from build123d import *

# Parameters (mm, degrees)
F1_DEPTH = 1750
F2_R     = 4
F3_R     = 2


with BuildPart() as f1:
    # F0 (on Front) → F1 (new body)
    with BuildSketch(Plane.XZ):
        Polygon((0, 0), (-20, 0), (-20, -10), (-10, -10), (-10, -75), (0, -75), align=None)
    extrude(amount=F1_DEPTH)

    # F2
    f2_edges = [f1.edges().sort_by_distance(p)[0] for p in [
        (0, -875, 0),
    ]]
    fillet(f2_edges, radius=F2_R)

    # F3
    f3_edges = [f1.edges().sort_by_distance(p)[0] for p in [
        (-10, -875, -10),
    ]]
    fillet(f3_edges, radius=F3_R)


solid = f1.part
Geometry check sheet. Reference: the model listing, model coordinates, mm. A direction names the side the tool comes from. Coordinates: 2 decimals unless noted, no trailing zeros. Loops run counter-clockwise (first coordinate to the right, second up) from the corner with the lowest first, then second, coordinate; pieces in that order, holes last. Notation, with made-up numbers: (80, 61) - (122, 61) arc R29 cw to (122, 100) - close; hole circle Ø2 at (65, 79). An arc over 180 degrees is marked (long way). Use one line per item in the form item = value. Start each with the question number.
Item 1: Section check C-C, the plane x = -15.5. Enter the section's corners in (y, z), and give its area (3 significant figures).
Item 2: Section check B-B, the plane z = -50. Enter the section's corners in (x, y).
Item 3: Tool access check on faces 1 (the face through (-10, -863, -43)), 2 (the face through (0, -863, -40)). Record the directions out of +Z, -Z, +X, -X, +Y, -Y that give a thin tool (end or side, any length) a straight path to the whole face; none if there is none.
Item 4: Gauge pin test, flat ends, axial feed: pin 1 (2.5 mm diameter, centred on x = -17.5, y = -802.5, fed in from -Z); pin 2 (4 mm diameter, centred on x = -13.5, z = -32.5, fed in from -Y); pin 3 (8 mm diameter, centred on y = -351, z = -39, fed in from -X). Record the tip position at first contact, or that the pin passes through.
Item 5: Section check A-A, the plane y = -1145.5. Enter the section's corners in (x, z).
Item 6: Thickness scan on probe 1 along Z at (x, y) = (-17.75, -340); probe 2 along X at (y, z) = (-1159, -11). Record the ranges inside material, lowest first.
Computed:
q1.outline = (-1750, -10) - (0, -10) - (0, 0) - (-1750, 0) - close
q1.area = 17,500 mm2
q2.outline = (-10, -1750) - (0, -1750) - (0, 0) - (-10, 0) - close
q3.face_1 = -Z, -X, +Y, -Y
q3.face_2 = +Z, -Z, +X, +Y, -Y
q4.pin_1 = -10
q4.pin_2 = through
q4.pin_3 = -10
q5.outline = (-20, -10) - (-12, -10) arc R2 cw to (-10, -12) - (-10, -75) - (0, -75) - (0, -4) arc R4 ccw to (-4, 0) - (-20, 0) - close
q6.probe_1 = -10 to 0
q6.probe_2 = -10.27 to 0
